Design review of the part built by this model. Coordinates are the model's own, in mm. Round coordinates to 2 decimals unless told otherwise and drop trailing zeros. Order: outer loops, then holes, each group sorted by start corner. A loop starts at its lowest first (then second) coordinate and runs counter-clockwise, first axis right, second up. Notation, with made-up numbers: M 69.25,-6 L 114.25,-6 A19 ccw 114.25,11 Z; hole C 30,25 d2. An arc over 180 degrees is marked long. Write each question's results on one line, items separated by ' | '. Start each with the question number.
Item 1: Wall thickness on line 1 (Y direction, x = -9, z = 2.2); line 2 (Y direction, x = -11.25, z = 1.15); line 3 (Y direction, x = -17.5, z = 1.6): over which ranges is each line inside the solid? List them lowest first. Write a range as [from, to].
Item 2: Take a section at A-A, the plane y = 99. Write out the cut boundary in (x, z), plus the area to 3 significant figures.
Item 3: Clearance check with flat-ended pins moving along their axes: pin 1 (1.5 mm diameter, centred on x = -16.5, z = 1, fed in from -Y); pin 2 (0.9 mm diameter, centred on y = 4.5, z = 1.5, fed in from -X); pin 3 (1.5 mm diameter, centred on y = 5, z = 1.5, fed in from +X). State where each tip first meets the part, or that it passes through.
Item 4: Take a section at B-B, the plane y = 28.5. Write out the cut boundary in (x, z), plus the area to 3 significant figures.
Autodesk Inventor part; units mm, degrees
ref_plane "YZ Plane" through (0, 0, 0) normal (1, 0, 0) x (0, 1, 0)
ref_plane "XZ Plane" through (0, 0, 0) normal (0, 1, 0) x (-1, 0, 0)
ref_plane "XY Plane" through (0, 0, 0) normal (0, 0, 1) x (1, 0, 0)
sketch "草圖1" plane through (0, 0, 0) normal (0, 0, 1) x (1, 0, 0)
  arc A0 (-7.5, 147.4544) -> (-7.5, 136.5456) centre (-10, 142) ccw construction
  arc A1 (-10, 4.5) -> (1.3043, 31.8231) centre (-10, 20.5) ccw
  line L0 (-10, 20.5) -> (-10, 4.5) construction
  line L1 (-10, 20.5) -> (-10, 48.1702) construction
  line L2 (-10, 8.3) -> (-10, 4.5)
  line L3 (-7.5, 284) -> (-22.5, 284)
  line L4 (-22.5, 284) -> (-22.5, 48.1702)
  line L5 (-22.5, 48.1702) -> (-10, 48.1702) construction
  line L6 (-7.5, 36.5) -> (-7.5, 53.0538) construction
  line L7 (-7.5, 36.5) -> (-7.5, 36.3035) construction
  line L8 (-10, 48.1702) -> (-10, 32.7) construction
  line L9 (-10, 32.7) -> (-22.5, 32.7)
  line L10 (-22.5, 32.7) -> (-22.5, 48.1702)
  arc A2 (-7.5, 53.0538) -> (1.3043, 31.8231) centre (22.5, 53.0538) ccw
  arc A3 (1.3043, 31.8231) -> (-7.5, 36.3035) centre (-10, 20.5) ccw construction
  line L11 (-7.5, 53.0538) -> (-7.5, 64.05)
  line L12 (-7.5, 219.95) -> (-15, 219.95)
  line L13 (-15, 219.95) -> (-15, 217)
  line L14 (-15, 217) -> (-7.5, 217)
  line L15 (-7.5, 217) -> (-7.5, 219.95) construction
  line L16 (-7.5, 174.95) -> (-15, 174.95)
  line L17 (-15, 174.95) -> (-15, 172)
  line L18 (-15, 172) -> (-7.5, 172)
  line L19 (-7.5, 172) -> (-7.5, 174.95) construction
  line L20 (-7.5, 112) -> (-15, 112)
  line L21 (-15, 112) -> (-15, 109.05)
  line L22 (-15, 109.05) -> (-7.5, 109.05)
  line L23 (-7.5, 109.05) -> (-7.5, 112) construction
  line L24 (-7.5, 67) -> (-15, 67)
  line L25 (-15, 67) -> (-15, 64.05)
  line L26 (-15, 64.05) -> (-7.5, 64.05)
  line L27 (-7.5, 64.05) -> (-7.5, 67) construction
  line L28 (-7.5, 217) -> (-7.5, 219.95) construction
  line L29 (-7.5, 174.95) -> (-7.5, 217)
  line L30 (-7.5, 172) -> (-7.5, 174.95) construction
  line L31 (-7.5, 112) -> (-7.5, 172)
  line L32 (-7.5, 109.05) -> (-7.5, 112) construction
  line L33 (-7.5, 67) -> (-7.5, 109.05)
  line L34 (-7.5, 64.05) -> (-7.5, 67) construction
  line L35 (-7.5, 219.95) -> (-7.5, 284)
  arc A4 (-10, 8.3) -> (-10, 32.7) centre (-10, 20.5) ccw
  arc A5 (-12.7221, 32.7) -> (-10, 8) centre (-10, 20.5) ccw construction
  line L36 (-10, 4.5) -> (6, 4.5)
  line L37 (6, 4.5) -> (6, 0)
  line L38 (6, 0) -> (-10, 0)
  line L39 (-10, 0) -> (-10, 4.5)
  line L40 (6, 4.5) -> (6, 20.5)
  point P0 (0, 0)
  dimension "d12" = 16
  dimension "d13" = 180
  dimension "d14" = 15
  dimension "d16" = 60
  dimension "d17" = 30
  dimension "d18" = 75
  dimension "d19" = 30
  dimension "d20" = 75
  dimension "d21" = 2.95
  dimension "d22" = 2.95
  dimension "d23" = 2.95
  dimension "d24" = 2.95
  dimension "d25" = 7.5
  dimension "d30" = 24.4
  dimension "d31" = 25
  dimension "d32" = 4.5
  dimension "d38" = 284
extrude "擠出1" add sketch "草圖1" along normal blind 3
sketch "草圖3" plane through (0, 0, 3) normal (0, 0, 1) x (1, 0, 0)
  line L0 (-10, 8.3) -> (-10, 0)
  line L1 (-10, 5.9) -> (-2, 5.9)
  line L2 (-2, 5.9) -> (-2, 3)
  line L3 (-2, 3) -> (-10, 3)
  line L4 (-10, 3) -> (-10, 5.9)
  line L5 (-10, 0) -> (6, 0)
  line L6 (-2, 5.9) -> (6, 5.9)
  line L7 (6, 5.9) -> (6, 3)
  line L8 (6, 3) -> (-2, 3)
  line L9 (-2, 3) -> (-2, 5.9)
  line L10 (6, 0) -> (6, 20.5)
  point P0 (0, 0)
  dimension "d33" = 2.9
  dimension "d34" = 3
  dimension "d39" = 8
extrude "擠出2" cut sketch "草圖3" against normal up to surface (3 mm away) contours L6 L7 L8 L2
sketch "草圖4" plane through (0, 0, 3) normal (0, 0, 1) x (1, 0, 0)
  line L0 (-22.5, 284) -> (-22.5, 32.7)
  line L1 (-22.5, 281) -> (-16.5, 281)
  line L2 (-16.5, 281) -> (-16.5, 278.1)
  line L3 (-16.5, 278.1) -> (-22.5, 278.1)
  line L4 (-22.5, 278.1) -> (-22.5, 281)
  line L5 (-7.5, 284) -> (-22.5, 284)
  point P0 (0, 0)
  dimension "d40" = 3
  dimension "d41" = 2.9
  dimension "d42" = 6
extrude "擠出3" cut sketch "草圖4" against normal up to surface (3 mm away)
sketch "草圖5" plane through (0, 0, 3) normal (0, 0, 1) x (1, 0, 0)
  line L0 (-16.5, 278.1) -> (-22.5, 278.1)
  line L1 (-22.5, 278.1) -> (-22.5, 32.7)
  line L2 (-22.5, 32.7) -> (-10, 32.7)
  arc A0 (-10, 8.3) -> (-10, 32.7) centre (-10, 20.5) ccw
  line L3 (-10, 8.3) -> (-10, 0)
  line L4 (-10, 0) -> (6, 0)
  line L5 (6, 0) -> (6, 3)
  line L6 (6, 3) -> (-2, 3)
  line L7 (-2, 3) -> (-2, 5.9)
  line L8 (-2, 5.9) -> (6, 5.9)
  line L9 (6, 5.9) -> (6, 20.5)
  arc A1 (6, 20.5) -> (1.3043, 31.8231) centre (-10, 20.5) ccw
  arc A2 (-7.5, 53.0538) -> (1.3043, 31.8231) centre (22.5, 53.0538) ccw
  line L10 (-7.5, 53.0538) -> (-7.5, 64.05)
  line L11 (-7.5, 64.05) -> (-15, 64.05)
  line L12 (-15, 64.05) -> (-15, 67)
  line L13 (-15, 67) -> (-7.5, 67)
  line L14 (-7.5, 67) -> (-7.5, 109.05)
  line L15 (-7.5, 109.05) -> (-15, 109.05)
  line L16 (-15, 109.05) -> (-15, 112)
  line L17 (-15, 112) -> (-7.5, 112)
  line L18 (-7.5, 112) -> (-7.5, 172)
  line L19 (-7.5, 172) -> (-15, 172)
  line L20 (-15, 172) -> (-15, 174.95)
  line L21 (-15, 174.95) -> (-7.5, 174.95)
  line L22 (-7.5, 174.95) -> (-7.5, 217)
  line L23 (-7.5, 217) -> (-15, 217)
  line L24 (-15, 217) -> (-15, 219.95)
  line L25 (-15, 219.95) -> (-7.5, 219.95)
  line L26 (-7.5, 219.95) -> (-7.5, 284)
  line L27 (-7.5, 284) -> (-22.5, 284)
  line L28 (-22.5, 284) -> (-22.5, 281)
  line L29 (-22.5, 281) -> (-16.5, 281)
  line L30 (-16.5, 281) -> (-16.5, 278.1)
  point P0 (0, 0)
equation "\"d25\" = 0.5 * d14"
properties part number "chassis_1_5"
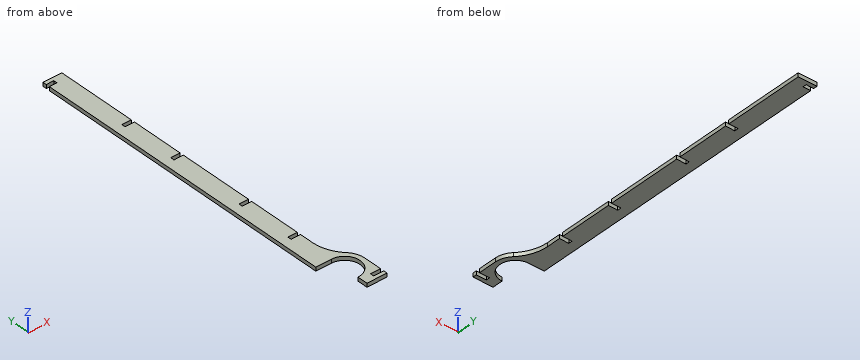
Results list:
1) line 1: [0, 8.34], [32.66, 64.05], [67, 109.05], [112, 172], [174.95, 217], [219.95, 284] | line 2: [32.7, 64.05], [67, 109.05], [112, 172], [174.95, 217], [219.95, 284] | line 3: [32.7, 278.1], [281, 284]
2) outline: M -22.5,0 L -7.5,0 L -7.5,3 L -22.5,3 Z | area: 45.0 mm²
3) pin 1: y = 32.7 | pin 2: x = -10 | pin 3: x = -2
4) outline: M -0.79,0 L 3.86,0 L 3.86,3 L -0.79,3 Z | area: 13.9 mm²
